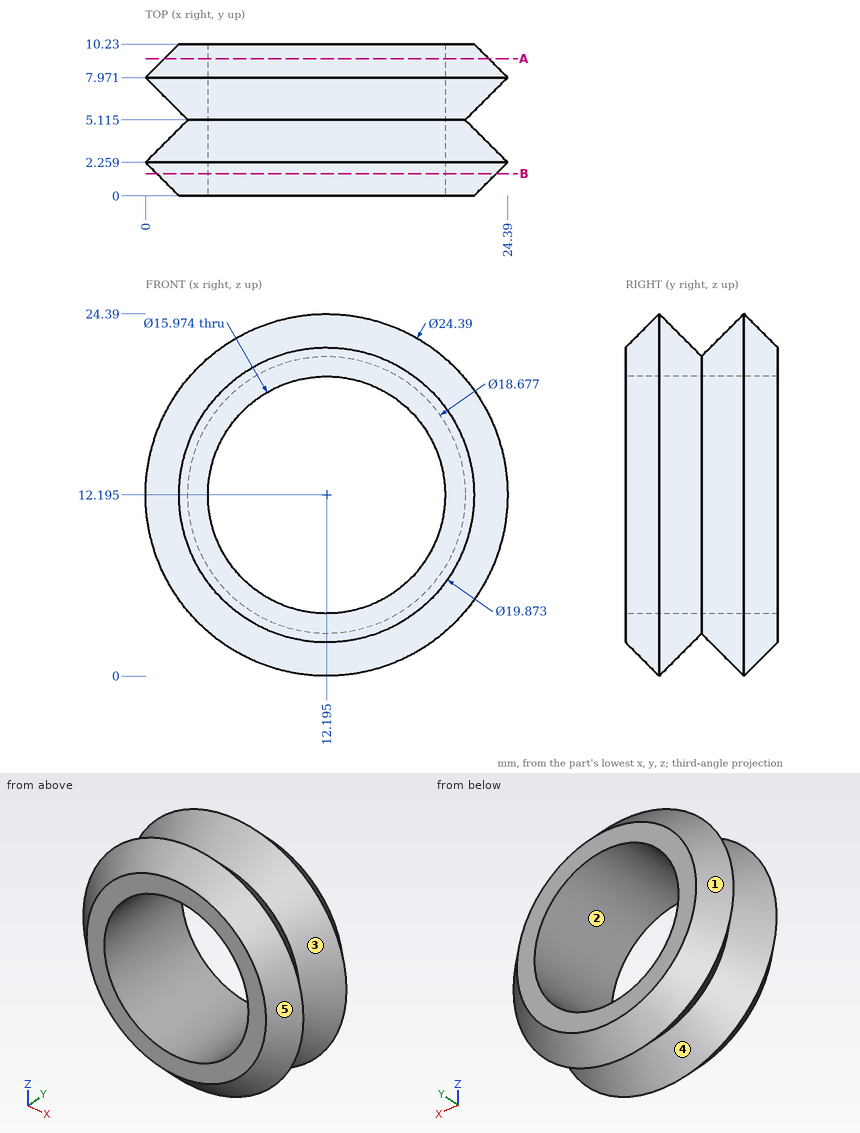
Check sheet for the drawn part. Datum: minimum x, y, z corner. Units: mm. A direction names the side the tool comes from. Round coordinates to 2 decimals unless told otherwise and drop trailing zeros. Order: outer loops, then holes, each group sorted by start corner. A loop starts at its lowest first (then second) coordinate and runs counter-clockwise, first axis right, second up. Notation, with made-up numbers: (1, 55.25) - (5, 55.25) arc R19 ccw to (5, 59.25) - close; hole circle Ø1 at (24, 2). An arc over 180 degrees is marked (long way). Use a Markdown table: item, result. Add a question column.
(1) Sectioned sample at B-B, the plane y = 1.5. Enter the section's corners in (x, z) (1 decimal).
(2) Tool access check on the marked faces 4 and 5. Record the directions out of +Z, -Z, +X, -X, +Y, -Y that give a thin tool (end or side, any length) a straight path to the whole face; none if there is none.
(3) Sectioned sample at A-A, the plane y = 9.25. Enter the section's corners in (x, z) (1 decimal).
(4) Material ranges on line 1 along X through (y, z) = (8.5, 9.75); line 2 along Y through (x, z) = (1, 9) (1 decimal); line 3 along X through (y, z) = (6.25, 16) (1 decimal), recorded low to high. Write a range as [from, to].
(5) Depth check by flat-ended pin: pin 1 (3 mm diameter, centred on x = 10.5, y = 3.5, fed in from +Z); pin 2 (13 mm diameter, centred on x = 12.195, z = 12.195, fed in from -Y); pin 3 (3 mm diameter, centred on x = 21, y = 3.5, fed in from -Z); pin 4 (4 mm diameter, centred on x = 7.5, y = 4, fed in from +Z). Enter the tip coordinate at first touch or a pass-through.
(6) Release check for a two-part mould opening along Y. For the marked faces 1, 2 and 3 record: pulls with the +Y half, pulls with the -Y half, needs draft (parallel to the pull), parting line crosses it, or undercut.
Answers below:
| question | item | result |
|---|---|---|
| 1 | outline | circle Ø22.9 at (12.2, 12.2); hole circle Ø16 at (12.2, 12.2) |
| 2 | face 4 | none |
| 2 | face 5 | -Y |
| 3 | outline | circle Ø21.8 at (12.2, 12.2); hole circle Ø16 at (12.2, 12.2) |
| 4 | line 1 | [0.79, 4.59], [19.8, 23.6] |
| 4 | line 2 | [1.7, 2.8], [7.4, 8.5] |
| 4 | line 3 | [2.4, 5.2], [19.2, 22] |
| 5 | pin 1 | z = 24.36 |
| 5 | pin 2 | through |
| 5 | pin 3 | z = 2.96 |
| 5 | pin 4 | z = 23.81 |
| 6 | face 1 | pulls with the +Y half |
| 6 | face 2 | needs draft |
| 6 | face 3 | undercut |
